CAD build for the part. Positions are in the model's coordinates, mm. A direction names the side the tool comes from. Round coordinates to 2 decimals unless told otherwise and drop trailing zeros.
from build123d import *

# Parameters (mm, degrees)
PAD001_DEPTH = 1.6
FILLET001_R  = 0.75
PAD_DEPTH    = 1.6
FILLET_R     = 0.75
BOX_W        = 30
BOX_H        = 8
BOX_DEPTH    = 30
FILLET002_R  = 1
FILLET003_R  = 1
FILLET004_R  = 1
FILLET005_R  = 1


with BuildPart() as fillet001:
    # Sketch001 → Pad001 (new body)
    with BuildSketch(Plane(origin=(0, 0, 0.8), x_dir=(0, 1, 0), z_dir=(1, 0, 0))):
        Polygon((11.3125, 0.040257), (8.667595, -14.959743), (0.040255, -14.959743), (0.040255, 15.040257), (8.667595, 15.040257), align=None)
    extrude(amount=PAD001_DEPTH)

    # Fillet001
    fillet001_edges = [fillet001.edges().sort_by_distance(p)[0] for p in [
        (1.6, 9.990048, 8.340257),
        (0, 9.990048, 8.340257),
        (1.6, 9.990048, -6.659743),
        (0, 9.990048, -6.659743),
    ]]
    fillet(fillet001_edges, radius=FILLET001_R)


with BuildPart() as fusion:
    # Sketch → Pad (new body)
    with BuildSketch(Plane(origin=(0.8, 0, 0), x_dir=(1, 0, 0), z_dir=(0, 0, 1))):
        Polygon((-15, 0), (15, 0), (15, 10), (0, 11.304791), (-15, 10), align=None)
    extrude(amount=PAD_DEPTH)

    # Fillet
    fillet_edges = [fusion.edges().sort_by_distance(p)[0] for p in [
        (8.3, 10.652395, 0),
        (8.3, 10.652395, 1.6),
        (-6.7, 10.652396, 1.6),
        (-6.7, 10.652396, 0),
    ]]
    fillet(fillet_edges, radius=FILLET_R)

    # Fusion: union Fillet001
    add(fillet001.part)


with BuildPart() as fillet005:
    # Box → Box (new body)
    with BuildSketch(Plane(origin=(-14.2, 8, -14.2), x_dir=(1, 0, 0), z_dir=(0, 0, 1))):
        with Locations((15, 4)):
            Rectangle(BOX_W, BOX_H)
    extrude(amount=BOX_DEPTH)

    # Cut: cut Fusion
    add(fusion.part, mode=Mode.SUBTRACT)

    # Fillet002
    fillet002_edges = [fillet005.edges().sort_by_distance(p)[0] for p in [
        (15.8, 8, -7.1),
    ]]
    fillet(fillet002_edges, radius=FILLET002_R)

    # Fillet003
    fillet003_edges = [fillet005.edges().sort_by_distance(p)[0] for p in [
        (15.8, 8, 8.7),
    ]]
    fillet(fillet003_edges, radius=FILLET003_R)

    # Fillet004
    fillet004_edges = [fillet005.edges().sort_by_distance(p)[0] for p in [
        (-14.2, 8, -7.1),
    ]]
    fillet(fillet004_edges, radius=FILLET004_R)

    # Fillet005
    fillet005_edges = [fillet005.edges().sort_by_distance(p)[0] for p in [
        (-14.2, 8, 8.7),
    ]]
    fillet(fillet005_edges, radius=FILLET005_R)


solid = fillet005.part
Item 1: Wall check: L1, parallel to X at y = 10, z = 3.5; L2, parallel to X at y = 8.5, z = 14.5. Give the ranges that are in metal, low to high.
Verdict:
L1: x = -14.2 to 0, 1.6 to 15.8
L2: x = -14.07 to 0.09, 1.51 to 15.67
Item 2: 3-axis set-ups, long thin cutter, end or side, ignore diameter. For faces 1 (the flat face through (1.6, 9, 6)), 2 (the flat face through (-7, 8, 9)): which of +Z, -Z, +X, -X, +Y, -Y reach the whole face in a straight line?
Verdict:
face 1: -Y
face 2: +Z, -Z, +X, -X, -Y
Item 3: Mould opens along X. For faces 3 (the flat face through (8, 8, 9)), 4 (the cylindrical face through (-6.9, 10.42, 1.374)), 5 (the flat face through (15.8, 12, 1)) say: released by +X, released by -X, zero draft, split by the parting line, or undercut.
Verdict:
face 3: zero draft
face 4: undercut
face 5: released by +X
